Read the model definition and answer for the solid it produces. Units are mm, in the model's axes. Face numbers are marked on the shaded views. A direction names the side the tool comes from. Give positions to 0.01 mm unless a question says otherwise; leave off trailing zeros. Write each loop counter-clockwise with the first axis right and the second up, starting at its lowest first coordinate (ties: lowest second). Pieces come first, ordered by that corner, then holes. Notation, with made-up numbers: (74.5, -23) -> (117.5, -23) arc R16 cw to (117.5, 7) -> close; hole circle Ø10 at (80, -32). An arc over 180 degrees is marked (long way). Use a Markdown table: item, result.
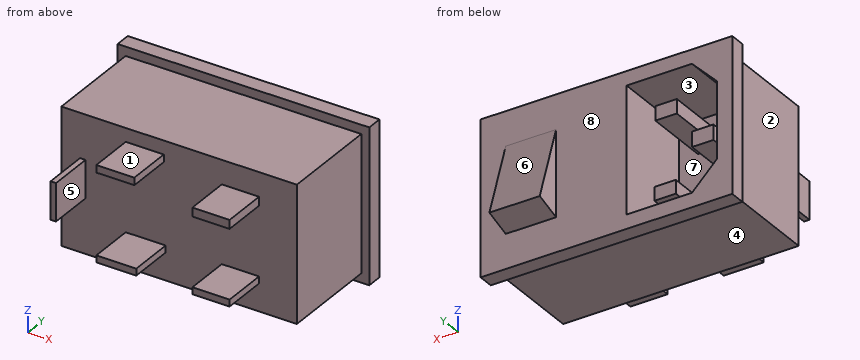
from build123d import *

# Parameters (mm, degrees)
SKETCH_1_W          = 50
SKETCH_1_H          = 30.6
EXTRUDE_1_DEPTH     = 3.1
SKETCH_2_W          = 46.8
SKETCH_2_H          = 27
EXTRUDE_2_DEPTH     = 19.7
CUT_EXTRUDE_1_DEPTH = 16
SKETCH_4_W          = 4.267620073
SKETCH_4_H          = 3.000670364
SKETCH_4_W_2        = 4.267620072
SKETCH_4_H_2        = 2.667262545
SKETCH_4_H_3        = 2.826910105
EXTRUDE_3_DEPTH     = 13
EXTRUDE_START       = -5
EXTRUDE_4_DEPTH     = 10
SKETCH_6_W          = 1.087762737
SKETCH_6_H          = 7.451174749
SKETCH_6_W_2        = 7.559951024
SKETCH_6_H_2        = 1.468479696
SKETCH_6_W_3        = 7.940667982
SKETCH_6_H_3        = 1.359703422
SKETCH_6_W_4        = 7.396786613
SKETCH_6_H_4        = 1.74042038
EXTRUDE_5_DEPTH     = 9


with BuildPart() as part:
    # 草图1 → 凸台-拉伸1 (new body)
    with BuildSketch(Plane(origin=(0, 0, 0), x_dir=(1, 0, 0), z_dir=(0, 1, 0))):
        Rectangle(SKETCH_1_W, SKETCH_1_H)
    extrude(amount=EXTRUDE_1_DEPTH)

    # 草图2 → 凸台-拉伸2 (add)
    with BuildSketch(Plane.XZ):
        Rectangle(SKETCH_2_W, SKETCH_2_H)
    extrude(amount=EXTRUDE_2_DEPTH)

    # 草图3 → 切除-拉伸1 (cut)
    with BuildSketch(Plane(origin=(0, 3.1, 0), x_dir=(1, 0, 0), z_dir=(0, 1, 0))):
        Polygon((-17, 12.5), (-4, 12.5), (-4, -12.5), (-17, -12.5), (-22, -7.5), (-22, 7.5), align=None)
    extrude(amount=-CUT_EXTRUDE_1_DEPTH, mode=Mode.SUBTRACT)

    # 草图4 → 凸台-拉伸3 (add)
    with BuildSketch(Plane(origin=(0, -12.9, 0), x_dir=(1, 0, 0), z_dir=(0, 1, 0))):
        with Locations((-17.186695536, 0)):
            Rectangle(SKETCH_4_W, SKETCH_4_H)
        with Locations((-9.718360408, 8.168491546)):
            Rectangle(SKETCH_4_W_2, SKETCH_4_H_2)
        with Locations((-9.918405099, -7.368312782)):
            Rectangle(SKETCH_4_W_2, SKETCH_4_H_3)
    extrude(amount=EXTRUDE_3_DEPTH)

    # 草图5 → 凸台-拉伸4 (add)
    with BuildSketch(Plane(origin=(25, 0, 0), x_dir=(0, 0, -1), z_dir=(1, 0, 0)).offset(EXTRUDE_START)):
        Polygon((-8.5, 3.1), (6.873863542, 8.1), (8.5, 3.1), align=None)
    extrude(amount=-EXTRUDE_4_DEPTH)

    # 草图6 → 凸台-拉伸5 (add)
    with BuildSketch(Plane.XZ.offset(19.7)):
        with Locations((-19.144624175, 0.978986463)):
            Rectangle(SKETCH_6_W, SKETCH_6_H)
        with Locations((-6.825711176, 10.061805319)):
            Rectangle(SKETCH_6_W_2, SKETCH_6_H_2)
        with Locations((-6.635352697, -7.396786613)):
            Rectangle(SKETCH_6_W_3, SKETCH_6_H_3)
        with Locations((12.182942656, 7.859085776)):
            Rectangle(SKETCH_6_W_4, SKETCH_6_H_4)
        with Locations((12.182942656, -7.396786613)):
            Rectangle(SKETCH_6_W_4, SKETCH_6_H_3)
    extrude(amount=EXTRUDE_5_DEPTH)


solid = part.part
Item 1: Straight lines are drawn through the part: line 1 along X through (y, z) = (-10.5, 7); line 2 along Z through (x, y) = (-6.5, -24); line 3 along X through (y, z) = (-3, 4). For each, find the intervals that lie inside material, in ascending order. Write a range as [from, to].
Return value:
| item | result |
|---|---|
| line 1 | [-23.4, -22], [-12.05, -7.78], [-4, 23.4] |
| line 2 | [-8.08, -6.72], [9.33, 10.8] |
| line 3 | [-23.4, -22], [-4, 23.4] |
Item 2: A cutting plane is placed at A-A (y = -23). Give the vertices of the cut face in (x, z).
Return value:
| item | result |
|---|---|
| outline | (-19.69, -2.75) -> (-18.6, -2.75) -> (-18.6, 4.7) -> (-19.69, 4.7) -> close; (-10.61, -8.08) -> (-2.67, -8.08) -> (-2.67, -6.72) -> (-10.61, -6.72) -> close; (-10.61, 9.33) -> (-3.05, 9.33) -> (-3.05, 10.8) -> (-10.61, 10.8) -> close; (8.48, -8.08) -> (15.88, -8.08) -> (15.88, -6.72) -> (8.48, -6.72) -> close; (8.48, 6.99) -> (15.88, 6.99) -> (15.88, 8.73) -> (8.48, 8.73) -> close |
Item 3: Each of these flat-tipped pins is pushed along its axis until it touches: P1, Ø3, axis at y = -9.5, z = -3.5, coming from the +X side; P2, Ø2, axis at x = -9.5, y = -5.5, coming from the -Z side; P3, Ø1.4, axis at x = -9.5, z = 7.5, coming from the +Y side. Where does it stop, or does it pass through?
Return value:
| item | result |
|---|---|
| P1 | x = 23.4 |
| P2 | z = -13.5 |
| P3 | y = 0.1 |
Item 4: A cutting plane is placed at D-D (y = 1). Give the vertices of the cut face in (x, z).
Return value:
| item | result |
|---|---|
| outline | (-25, -15.3) -> (25, -15.3) -> (25, 15.3) -> (-25, 15.3) -> close; hole (-22, -7.5) -> (-17, -12.5) -> (-4, -12.5) -> (-4, 12.5) -> (-17, 12.5) -> (-22, 7.5) -> close |
Item 5: A cutting plane is placed at B-B (y = -3). Give the vertices of the cut face in (x, z), then the cut area to 3 significant figures.
Return value:
| item | result |
|---|---|
| outline | (-23.4, -13.5) -> (23.4, -13.5) -> (23.4, 13.5) -> (-23.4, 13.5) -> close; (-19.32, -1.5) -> (-15.05, -1.5) -> (-15.05, 1.5) -> (-19.32, 1.5) -> close; (-12.05, 5.95) -> (-7.78, 5.95) -> (-7.78, 8.78) -> (-12.05, 8.78) -> close; (-11.85, -9.5) -> (-7.58, -9.5) -> (-7.58, -6.83) -> (-11.85, -6.83) -> close; hole (-22, -7.5) -> (-17, -12.5) -> (-4, -12.5) -> (-4, 12.5) -> (-17, 12.5) -> (-22, 7.5) -> close |
| area | 875 mm^2 |
Item 6: A cutting plane is placed at C-C (x = 12.5). Give the vertices of the cut face in (y, z).
Return value:
| item | result |
|---|---|
| outline | (-28.7, -8.08) -> (-19.7, -8.08) -> (-19.7, -13.5) -> (0, -13.5) -> (0, -15.3) -> (3.1, -15.3) -> (3.1, -8.5) -> (8.1, -6.87) -> (3.1, 8.5) -> (3.1, 15.3) -> (0, 15.3) -> (0, 13.5) -> (-19.7, 13.5) -> (-19.7, 8.73) -> (-28.7, 8.73) -> (-28.7, 6.99) -> (-19.7, 6.99) -> (-19.7, -6.72) -> (-28.7, -6.72) -> close |
Item 7: A tool of negligible diameter and unlimited length cuts with its end or side. For the marked faces 1, 2, 3, 4 and 5, from which of +Z, -Z, +X, -X, +Y, -Y can it reach the whole face along a straight path? Write none if from no direction.
Return value:
| item | result |
|---|---|
| face 1 | +Z, +X, -X, -Y |
| face 2 | +Z, -Z, -X, -Y |
| face 3 | +Y |
| face 4 | -Z, +X, -X, -Y |
| face 5 | +Z, -Z, +X, -Y |
Item 8: For a pull along Z with two mould halves and no side action, classify the marked faces 6, 7 and 8 as +Z half, -Z half, draft (parallel to the pull), parting line (faces both ways), or undercut.
Return value:
| item | result |
|---|---|
| face 6 | +Z half |
| face 7 | undercut |
| face 8 | draft |
